Here's how the part is built. I have some questions about the finished solid (model axes, mm). Face numbers are marked on the shaded views. Coordinates: 2 decimals unless noted, no trailing zeros. Write each loop counter-clockwise with the first axis right and the second up, starting at its lowest first coordinate (ties: lowest second). Pieces come first, ordered by that corner, then holes.
```python
from build123d import *

# Parameters (mm, degrees)
F1_DEPTH  = 1
F2_DEPTH  = 14
F4_DEPTH  = 13
F7_DEPTH  = 18
F10_DEPTH = 13
F13_DEPTH = 1.5875
F16_DEPTH = 1.5
F18_R     = 1
F19_DEPTH = 10
F21_R     = 1.5
F22_DEPTH = 2
F24_W     = 7
F24_H     = 7
F25_DEPTH = 3
F27_R     = 1
F28_DEPTH = 9


with BuildPart() as f1:
    # F0 (on Front) → F1 (new body)
    with BuildSketch(Plane.XZ):
        with BuildLine():
            Line((141, 98), (-141, 98))
            ThreePointArc((-141, 98), (-144.535534, 96.535534), (-146, 93))
            Line((-146, 93), (-146, -93))
            ThreePointArc((-146, -93), (-144.535534, -96.535534), (-141, -98))
            Line((-141, -98), (141, -98))
            ThreePointArc((141, -98), (144.535534, -96.535534), (146, -93))
            Line((146, -93), (146, 93))
            ThreePointArc((146, 93), (144.535534, 96.535534), (141, 98))
        make_face()
        with BuildLine():
            ThreePointArc((-125, 76.5), (-124.12132, 78.62132), (-122, 79.5))
            Line((-122, 79.5), (122, 79.5))
            ThreePointArc((122, 79.5), (124.12132, 78.62132), (125, 76.5))
            Line((125, 76.5), (125, -76.5))
            ThreePointArc((125, -76.5), (124.12132, -78.62132), (122, -79.5))
            Line((122, -79.5), (-122, -79.5))
            ThreePointArc((-122, -79.5), (-124.12132, -78.62132), (-125, -76.5))
            Line((-125, -76.5), (-125, 76.5))
        make_face(mode=Mode.SUBTRACT)
        with BuildLine():
            Line((122, 79.5), (-122, 79.5))
            ThreePointArc((-122, 79.5), (-124.12132, 78.62132), (-125, 76.5))
            Line((-125, 76.5), (-125, -76.5))
            ThreePointArc((-125, -76.5), (-124.12132, -78.62132), (-122, -79.5))
            Line((-122, -79.5), (122, -79.5))
            ThreePointArc((122, -79.5), (124.12132, -78.62132), (125, -76.5))
            Line((125, -76.5), (125, 76.5))
            ThreePointArc((125, 76.5), (124.12132, 78.62132), (122, 79.5))
        make_face()
        with BuildLine():
            ThreePointArc((-110.5, 59.5), (-109.62132, 61.62132), (-107.5, 62.5))
            Line((-107.5, 62.5), (107.5, 62.5))
            ThreePointArc((107.5, 62.5), (109.62132, 61.62132), (110.5, 59.5))
            Line((110.5, 59.5), (110.5, -59.5))
            ThreePointArc((110.5, -59.5), (109.62132, -61.62132), (107.5, -62.5))
            Line((107.5, -62.5), (-107.5, -62.5))
            ThreePointArc((-107.5, -62.5), (-109.62132, -61.62132), (-110.5, -59.5))
            Line((-110.5, -59.5), (-110.5, 59.5))
        make_face(mode=Mode.SUBTRACT)
    extrude(amount=-F1_DEPTH)

    # F0 (on Front) → F2 (join)
    with BuildSketch(Plane.XZ):
        with BuildLine():
            Line((141, 98), (-141, 98))
            ThreePointArc((-141, 98), (-144.535534, 96.535534), (-146, 93))
            Line((-146, 93), (-146, -93))
            ThreePointArc((-146, -93), (-144.535534, -96.535534), (-141, -98))
            Line((-141, -98), (141, -98))
            ThreePointArc((141, -98), (144.535534, -96.535534), (146, -93))
            Line((146, -93), (146, 93))
            ThreePointArc((146, 93), (144.535534, 96.535534), (141, 98))
        make_face()
        with BuildLine():
            ThreePointArc((-125, 76.5), (-124.12132, 78.62132), (-122, 79.5))
            Line((-122, 79.5), (122, 79.5))
            ThreePointArc((122, 79.5), (124.12132, 78.62132), (125, 76.5))
            Line((125, 76.5), (125, -76.5))
            ThreePointArc((125, -76.5), (124.12132, -78.62132), (122, -79.5))
            Line((122, -79.5), (-122, -79.5))
            ThreePointArc((-122, -79.5), (-124.12132, -78.62132), (-125, -76.5))
            Line((-125, -76.5), (-125, 76.5))
        make_face(mode=Mode.SUBTRACT)
    extrude(amount=-F2_DEPTH)


with BuildPart() as f4:
    # F3 (on face) → F4 (new body)
    with BuildSketch(Plane(origin=(0, 14, 0), x_dir=(-1, 0, 0), z_dir=(0, 1, 0))):
        with BuildLine():
            ThreePointArc((50, 92.5), (49.12132, 94.62132), (47, 95.5))
            Line((47, 95.5), (-47, 95.5))
            ThreePointArc((-47, 95.5), (-49.12132, 94.62132), (-50, 92.5))
            Line((-50, 92.5), (-50, 66.5))
            ThreePointArc((-50, 66.5), (-49.12132, 64.37868), (-47, 63.5))
            Line((-47, 63.5), (47, 63.5))
            ThreePointArc((47, 63.5), (49.12132, 64.37868), (50, 66.5))
            Line((50, 66.5), (50, 92.5))
        make_face()
    extrude(amount=-F4_DEPTH)


with BuildPart() as f1_1:
    add(f1.part)

    # F5: cut F4
    add(f4.part, mode=Mode.SUBTRACT)


with BuildPart() as f7:
    # F6 (on face) → F7 (new body)
    with BuildSketch(Plane.XY.offset(-79.5)):
        with BuildLine():
            Line((1.5, 17), (-1.5, 17))
            Line((-1.5, 17), (-1.5, 12.5))
            ThreePointArc((-1.5, 12.5), (-1.06066, 11.43934), (0, 11))
            ThreePointArc((0, 11), (1.06066, 11.43934), (1.5, 12.5))
            Line((1.5, 12.5), (1.5, 17))
        make_face()
    extrude(amount=-F7_DEPTH)


with BuildPart() as f1_2:
    add(f1_1.part)

    # F8: cut F7
    add(f7.part, mode=Mode.SUBTRACT)


with BuildPart() as f10:
    # F9 (on face) → F10 (new body)
    with BuildSketch(Plane(origin=(0, 14, 0), x_dir=(-1, 0, 0), z_dir=(0, 1, 0))):
        with BuildLine():
            Line((-123.5, 56.5), (-125.5, 56.5))
            ThreePointArc((-125.5, 56.5), (-126.207107, 56.207107), (-126.5, 55.5))
            Line((-126.5, 55.5), (-126.5, 11.5))
            ThreePointArc((-126.5, 11.5), (-126.207107, 10.792893), (-125.5, 10.5))
            Line((-125.5, 10.5), (-123.5, 10.5))
            Line((-123.5, 10.5), (-123.5, 56.5))
        make_face()
    extrude(amount=-F10_DEPTH)


with BuildPart() as f1_3:
    add(f1_2.part)

    # F11: cut F10
    add(f10.part, mode=Mode.SUBTRACT)


with BuildPart() as f13:
    # F12 (on face) → F13 (new body)
    with BuildSketch(Plane(origin=(0, 14, 0), x_dir=(-1, 0, 0), z_dir=(0, 1, 0))):
        with BuildLine():
            Line((-140.5, -31.5), (-131.5, -31.5))
            ThreePointArc((-131.5, -31.5), (-129.37868, -30.62132), (-128.5, -28.5))
            Line((-128.5, -28.5), (-128.5, 7.5))
            ThreePointArc((-128.5, 7.5), (-129.37868, 9.62132), (-131.5, 10.5))
            Line((-131.5, 10.5), (-140.5, 10.5))
            ThreePointArc((-140.5, 10.5), (-142.62132, 9.62132), (-143.5, 7.5))
            Line((-143.5, 7.5), (-143.5, -28.5))
            ThreePointArc((-143.5, -28.5), (-142.62132, -30.62132), (-140.5, -31.5))
        make_face()
        with BuildLine():
            ThreePointArc((128.5, -28.5), (129.37868, -30.62132), (131.5, -31.5))
            Line((131.5, -31.5), (140.5, -31.5))
            ThreePointArc((140.5, -31.5), (142.62132, -30.62132), (143.5, -28.5))
            Line((143.5, -28.5), (143.5, 7.5))
            ThreePointArc((143.5, 7.5), (142.62132, 9.62132), (140.5, 10.5))
            Line((140.5, 10.5), (131.5, 10.5))
            ThreePointArc((131.5, 10.5), (129.37868, 9.62132), (128.5, 7.5))
            Line((128.5, 7.5), (128.5, -28.5))
        make_face()
    extrude(amount=-F13_DEPTH)


with BuildPart() as f1_4:
    add(f1_3.part)

    # F14: cut F13
    add(f13.part, mode=Mode.SUBTRACT)


with BuildPart() as f16:
    # F15 (on face) → F16 (new body)
    with BuildSketch(Plane(origin=(0, 12.4125, 0), x_dir=(-1, 0, 0), z_dir=(0, 1, 0))):
        with BuildLine():
            ThreePointArc((-131.5, -3.5), (-132.37868, -1.37868), (-134.5, -0.5))
            Line((-134.5, -0.5), (-137.5, -0.5))
            ThreePointArc((-137.5, -0.5), (-139.62132, -1.37868), (-140.5, -3.5))
            Line((-140.5, -3.5), (-140.5, -17.5))
            ThreePointArc((-140.5, -17.5), (-139.62132, -19.62132), (-137.5, -20.5))
            Line((-137.5, -20.5), (-134.5, -20.5))
            ThreePointArc((-134.5, -20.5), (-132.37868, -19.62132), (-131.5, -17.5))
            Line((-131.5, -17.5), (-131.5, -3.5))
        make_face()
        with BuildLine():
            Line((137.5, -0.5), (134.5, -0.5))
            ThreePointArc((134.5, -0.5), (132.37868, -1.37868), (131.5, -3.5))
            Line((131.5, -3.5), (131.5, -17.5))
            ThreePointArc((131.5, -17.5), (132.37868, -19.62132), (134.5, -20.5))
            Line((134.5, -20.5), (137.5, -20.5))
            ThreePointArc((137.5, -20.5), (139.62132, -19.62132), (140.5, -17.5))
            Line((140.5, -17.5), (140.5, -3.5))
            ThreePointArc((140.5, -3.5), (139.62132, -1.37868), (137.5, -0.5))
        make_face()
    extrude(amount=-F16_DEPTH)


with BuildPart() as f1_5:
    add(f1_4.part)

    # F17: cut F16
    add(f16.part, mode=Mode.SUBTRACT)


with BuildPart() as f19:
    # F18 (on face) → F19 (new body)
    with BuildSketch(Plane(origin=(0, 12.4125, 0), x_dir=(-1, 0, 0), z_dir=(0, 1, 0))):
        with Locations((-136, 5.5)):
            Circle(F18_R)
        with Locations((-136, -26.5)):
            Circle(F18_R)
        with Locations((136, 5.5)):
            Circle(F18_R)
        with Locations((136, -26.5)):
            Circle(F18_R)
    extrude(amount=-F19_DEPTH)


with BuildPart() as f1_6:
    add(f1_5.part)

    # F20: cut F19
    add(f19.part, mode=Mode.SUBTRACT)


with BuildPart() as f22:
    # F21 (on face) → F22 (new body)
    with BuildSketch(Plane(origin=(0, 12.4125, 0), x_dir=(-1, 0, 0), z_dir=(0, 1, 0))):
        with Locations((-136, 5.5)):
            Circle(F21_R)
        with Locations((-136, -26.5)):
            Circle(F21_R)
        with Locations((136, -26.5)):
            Circle(F21_R)
        with Locations((136, 5.5)):
            Circle(F21_R)
    extrude(amount=-F22_DEPTH)


with BuildPart() as f1_7:
    add(f1_6.part)

    # F23: cut F22
    add(f22.part, mode=Mode.SUBTRACT)


with BuildPart() as f25:
    # F24 (on face) → F25 (new body)
    with BuildSketch(Plane(origin=(0, 14, 0), x_dir=(-1, 0, 0), z_dir=(0, 1, 0))):
        with Locations((-68.5, 83)):
            Rectangle(F24_W, F24_H)
        with Locations((68.5, 83)):
            Rectangle(F24_W, F24_H)
        with Locations((-68.5, -83)):
            Rectangle(F24_W, F24_H)
        with Locations((68.5, -83)):
            Rectangle(F24_W, F24_H)
    extrude(amount=-F25_DEPTH)


with BuildPart() as f1_8:
    add(f1_7.part)

    # F26: cut F25
    add(f25.part, mode=Mode.SUBTRACT)


with BuildPart() as f28:
    # F27 (on face) → F28 (new body)
    with BuildSketch(Plane(origin=(0, 11, 0), x_dir=(-1, 0, 0), z_dir=(0, 1, 0))):
        with Locations((-68.5, 83)):
            Circle(F27_R)
        with Locations((68.5, 83)):
            Circle(F27_R)
        with Locations((-68.5, -83)):
            Circle(F27_R)
        with Locations((68.5, -83)):
            Circle(F27_R)
    extrude(amount=-F28_DEPTH)


with BuildPart() as f1_9:
    add(f1_8.part)

    # F29: cut F28
    add(f28.part, mode=Mode.SUBTRACT)


solid = f1_9.part
```
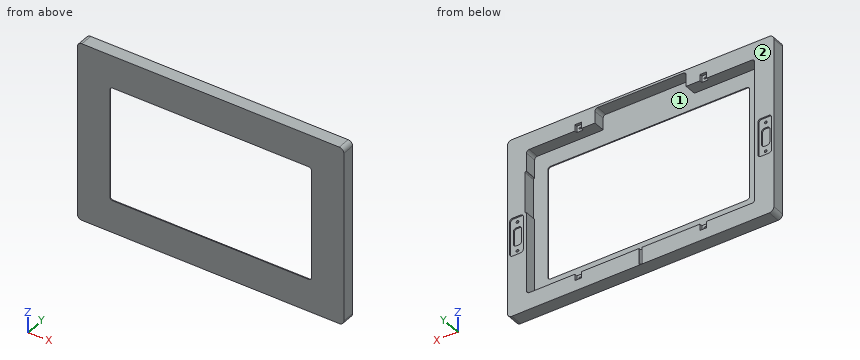
1) We'd pull the mould along Z, two halves only. Please class the marked faces 1 and 2: pulls with the +Z half, pulls with the -Z half, needs draft (parallel to the pull), parting line crosses it, or undercut.
Values follow:
face 1: undercut
face 2: needs draft
2) Will these pins go through, and if not, where does the flat tip stop? pin 1 (1 mm diameter, centred on x = 68.5, z = -83, fed in from +Y); pin 2 (2 mm diameter, centred on x = -68, z = 83.5, fed in from +Y); pin 3 (2.5 mm diameter, centred on x = 136, z = -26.5, fed in from +Y).
Values follow:
pin 1: stops at y = 2
pin 2: stops at y = 11
pin 3: stops at y = 10.41
3) I need wall thicknesses on probe 1 along Z at (x, y) = (136, 11.8); probe 2 along X at (y, z) = (5, 83); probe 3 along X at (y, z) = (9.75, 73.5). Which ranges of each line are inside material? Lowest first, please.
Values follow:
probe 1: z = -98 to -28, -25 to -20.5, -0.5 to 4, 7 to 98
probe 2: x = -146 to -69.5, -67.5 to -50, 50 to 67.5, 69.5 to 146
probe 3: x = -146 to -125, 125 to 146
4) Imagine slicing it at B-B on z = -41.5. Please give me the cut outline in (x, y).
Values follow:
outline: (-146, 0) - (-110.5, 0) - (-110.5, 1) - (-125, 1) - (-125, 14) - (-146, 14) - close; (110.5, 0) - (146, 0) - (146, 14) - (125, 14) - (125, 1) - (110.5, 1) - close
5) Imagine slicing it at A-A on z = 39.5. Please give me the cut outline in (x, y), then the cut area to 4 significant figures.
Values follow:
outline: (-146, 0) - (-110.5, 0) - (-110.5, 1) - (-125, 1) - (-125, 14) - (-146, 14) - close; (110.5, 0) - (146, 0) - (146, 14) - (126.5, 14) - (126.5, 1) - (110.5, 1) - close
area: 597.5 mm2
